Here's how the part is built. I have some questions about the finished solid (model axes, mm). Face numbers are marked on the shaded views. A direction names the side the tool comes from. Round coordinates to 2 decimals unless told otherwise and drop trailing zeros. Write each loop counter-clockwise with the first axis right and the second up, starting at its lowest first coordinate (ties: lowest second). Pieces come first, ordered by that corner, then holes. Notation, with made-up numbers: M -36.75,-23 L 7.25,-23 A27 ccw 7.25,-7 Z; hole C -4,3.5 d4. An arc over 180 degrees is marked long. Write item = value, one per line. Start each with the question number.
(1) On a 3-axis mill with a long thin cutter (end or side, diameter ignored), from which of +Z, -Z, +X, -X, +Y, -Y can I reach the whole of each face in a straight line? I mean the marked faces 5 and 6. Say none if no direction works.
(2) I want a section at A-A (z = 1.5). List the corners of the cut face in (x, y) for me.
(3) I want a section at C-C (x = 334). List the corners of the cut face in (y, z) for me, and give its area (3 significant figures).
(4) I need wall thicknesses on line 1 along X through (y, z) = (-226, 3); line 2 along X through (y, z) = (-224, 9.5); line 3 along Y through (x, z) = (334, 5). Which ranges of each line are inside material? Lowest first, please.
(5) I want a section at D-D (z = 4). List the corners of the cut face in (x, y) for me, and give its area (3 significant figures).
(6) I want a section at B-B (z = 6.25). List the corners of the cut face in (x, y) for me.
(7) Will these pins go through, and if not, where does the flat tip stop? pin 1 Ø4 at (x, y) = (333.5, -226) entering from +Z; pin 2 Ø9 at (x, y) = (332.73, -225.76) entering from +Z; pin 3 Ø3.5 at (x, y) = (309, -226) entering from +Z; pin 4 Ø1 at (y, z) = (-218.5, 7.5) entering from -X.
(8) If we mould it in two halves opening along Y, with no side actions, what happens to the marked faces 1, 2, 3 and 4? For each: released by +Y, released by -Y, zero draft, split by the parting line, or undercut.
```python
from build123d import *

# Parameters (mm, degrees)
SKETCH1_W           = 42.5
SKETCH1_H           = 27.5
BOSS_EXTRUDE1_DEPTH = 10
SKETCH2_R           = 5
CUT_EXTRUDE1_DEPTH  = 3
SKETCH3_W           = 4.2
SKETCH3_H           = 4.2
CUT_EXTRUDE2_DEPTH  = 5
SKETCH4_R           = 3.75
CUT_EXTRUDE3_DEPTH  = 7.5
FILLET1_R           = 10


with BuildPart() as part:
    # Sketch1 → Boss-Extrude1 (new body)
    with BuildSketch(Plane.XY):
        with Locations((325.175597792, -225.758680099)):
            Rectangle(SKETCH1_W, SKETCH1_H)
    extrude(amount=BOSS_EXTRUDE1_DEPTH)

    # Sketch2 → Cut-Extrude1 (cut)
    with BuildSketch(Plane.XY.offset(10)):
        with Locations((332.725597792, -225.758680099)):
            Circle(SKETCH2_R)
    extrude(amount=-CUT_EXTRUDE1_DEPTH, mode=Mode.SUBTRACT)

    # Sketch3 → Cut-Extrude2 (cut)
    with BuildSketch(Plane.XY.offset(10)):
        with Locations((308.025597792, -225.758680099)):
            Rectangle(SKETCH3_W, SKETCH3_H)
    extrude(amount=-CUT_EXTRUDE2_DEPTH, mode=Mode.SUBTRACT)

    # Sketch4 → Cut-Extrude3 (cut)
    with BuildSketch(Plane.XY.offset(10)):
        with Locations((332.725597792, -225.758680099)):
            Circle(SKETCH4_R)
    extrude(amount=-CUT_EXTRUDE3_DEPTH, mode=Mode.SUBTRACT)

    # Fillet1
    fillet1_edges = [part.edges().sort_by_distance(p)[0] for p in [
        (303.925597792, -212.008680099, 5),
        (303.925597792, -239.508680099, 5),
        (346.425597792, -239.508680099, 5),
        (346.425597792, -212.008680099, 5),
    ]]
    fillet(fillet1_edges, radius=FILLET1_R)


solid = part.part
```
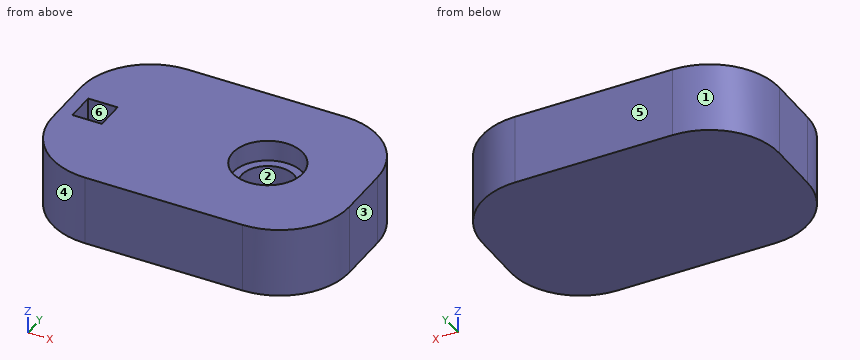
Returned:
q1.face_5 = +Z, -Z, +X, -X, +Y
q1.face_6 = +Z
q2.outline = M 303.93,-229.51 A10 ccw 313.93,-239.51 L 336.43,-239.51 A10 ccw 346.43,-229.51 L 346.43,-222.01 A10 ccw 336.43,-212.01 L 313.93,-212.01 A10 ccw 303.93,-222.01 Z
q3.outline = M -239.51,0 L -212.01,0 L -212.01,10 L -220.92,10 L -220.92,7 L -222.23,7 L -222.23,2.5 L -229.29,2.5 L -229.29,7 L -230.59,7 L -230.59,10 L -239.51,10 Z
q3.area = 214 mm²
q4.line_1 = 303.93 to 328.98, 336.47 to 346.43
q4.line_2 = 303.93 to 305.93, 310.13 to 328.05, 337.41 to 346.43
q4.line_3 = -239.51 to -229.29, -222.23 to -212.01
q5.outline = M 303.93,-229.51 A10 ccw 313.93,-239.51 L 336.43,-239.51 A10 ccw 346.43,-229.51 L 346.43,-222.01 A10 ccw 336.43,-212.01 L 313.93,-212.01 A10 ccw 303.93,-222.01 Z; hole C 332.73,-225.76 d7.5
q5.area = 1,040 mm²
q6.outline = M 303.93,-229.51 A10 ccw 313.93,-239.51 L 336.43,-239.51 A10 ccw 346.43,-229.51 L 346.43,-222.01 A10 ccw 336.43,-212.01 L 313.93,-212.01 A10 ccw 303.93,-222.01 Z; hole M 305.93,-227.86 L 310.13,-227.86 L 310.13,-223.66 L 305.93,-223.66 Z; hole C 332.73,-225.76 d7.5
q7.pin_1 = 2.5
q7.pin_2 = 7
q7.pin_3 = 10
q7.pin_4 = 304.39
q8.face_1 = released by +Y
q8.face_2 = undercut
q8.face_3 = zero draft
q8.face_4 = released by -Y
